from build123d import *

# Parameters (mm, degrees)
BOSS_EXTRUDE2_DEPTH = 2.5
BOSS_EXTRUDE3_DEPTH = 4


with BuildPart() as part:
    # Sketch1 → Boss-Extrude2 (new body)
    with BuildSketch(Plane(origin=(0, 0, 0), x_dir=(1, 0, 0), z_dir=(0, 1, 0))):
        Polygon((-52.914786993, 31.596385048), (-11.274786993, 31.596385048), (22.085213007, -6.979648962), (22.085213007, -27.403614952), (-52.914786993, -27.403614952), align=None)
    extrude(amount=BOSS_EXTRUDE2_DEPTH)

    # Sketch2 → Boss-Extrude3 (add)
    with BuildSketch(Plane(origin=(0, 2.5, 0), x_dir=(1, 0, 0), z_dir=(0, 1, 0))):
        Polygon((18.085213007, -23.403614952), (-48.914786993, -23.403614952), (-48.914786993, 27.596385048), (-13.10390193, 27.596385048), (18.085213007, -8.469333134), align=None)
        Polygon((14.085213007, -19.403614952), (-44.914786993, -19.403614952), (-44.914786993, 23.596385048), (-14.933016866, 23.596385048), (14.085213007, -9.959017305), align=None, mode=Mode.SUBTRACT)
    extrude(amount=BOSS_EXTRUDE3_DEPTH)


solid = part.part
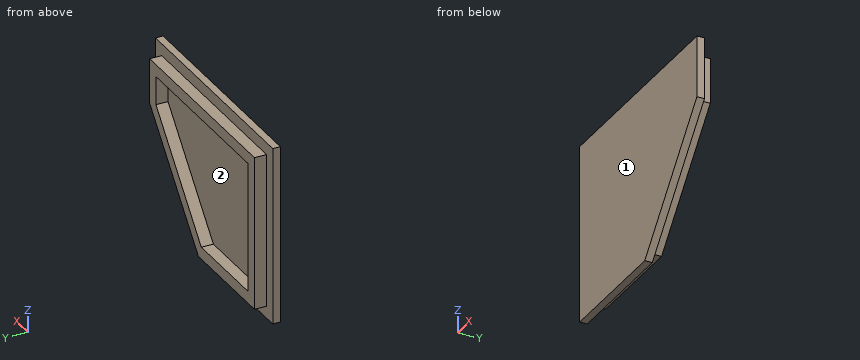
Geometry check sheet. Reference: the model listing, model coordinates, mm. Face numbers are marked on the shaded views. Give positions to 0.01 mm unless a question says otherwise; leave off trailing zeros. Write each loop counter-clockwise with the first axis right and the second up, starting at its lowest first coordinate (ties: lowest second). Pieces come first, ordered by that corner, then holes. Notation, with made-up numbers: M 86.5,80.25 L 116.5,80.25 A17 cw 116.5,96.25 Z; hole C 6.5,36 d2. An arc over 180 degrees is marked long. One line per question, with ' | ' between items.
1. Scan lines: line 1 along X through (y, z) = (4, 16); line 2 along Z through (x, y) = (-43.5, 4); line 3 along Y through (x, z) = (-9, -11). Record each from-to range of solid material in increasing order. Write a range as from..to.
Ans:
line 1: -48.91..-44.91, 14.09..18.09 | line 2: -27.6..-23.6, 19.4..23.4 | line 3: 0..2.5
2. Cross-section at D-D (y = 1.25). Enter the section's corners in (x, z), plus the area to 3 significant figures.
Ans:
outline: M -52.91,-31.6 L -11.27,-31.6 L 22.09,6.98 L 22.09,27.4 L -52.91,27.4 Z | area: 3,780 mm2
3. Cross-section at C-C (z = -10). Enter the section's corners in (x, y), plus the area to 3 significant figures.
Ans:
outline: M -52.91,0 L 7.4,0 L 7.4,2.5 L 2.11,2.5 L 2.11,6.5 L -3.18,6.5 L -3.18,2.5 L -44.91,2.5 L -44.91,6.5 L -48.91,6.5 L -48.91,2.5 L -52.91,2.5 Z | area: 188 mm2
4. Cross-section at A-A (y = 5.5). Enter the section's corners in (x, z).
Ans:
outline: M -48.91,-27.6 L -13.1,-27.6 L 18.09,8.47 L 18.09,23.4 L -48.91,23.4 Z; hole M -44.91,-23.6 L -14.93,-23.6 L 14.09,9.96 L 14.09,19.4 L -44.91,19.4 Z
5. Mould release check, pull along Z, two halves, no side actions. Record for the marked faces 1 and 2: released by +Z, released by -Z, zero draft, split by the parting line, or undercut.
Ans:
face 1: zero draft | face 2: undercut
6. Cross-section at B-B (x = -47). Enter the section's corners in (y, z), plus the area to 4 significant figures.
Ans:
outline: M 0,-31.6 L 2.5,-31.6 L 2.5,-27.6 L 6.5,-27.6 L 6.5,23.4 L 2.5,23.4 L 2.5,27.4 L 0,27.4 Z | area: 351.5 mm2
7. Gauge pin test, flat ends, axial feed: pin 1 (3 mm diameter, centred on y = 5, z = 15.5, fed in from -X); pin 2 (2 mm diameter, centred on x = -2, y = 5, fed in from +Z); pin 3 (1.2 mm diameter, centred on x = -31, y = 4, fed in from -Z). Record the tip position at first contact, or that the pin passes through.
Ans:
pin 1: x = -48.91 | pin 2: z = 23.4 | pin 3: z = -27.6
